from build123d import *
from build123d.topology import SkipClean

# Parameters (mm, degrees)
SKETCH1_R               = 107.5
BOSS_EXTRUDE1_DEPTH     = 5
BOSS_EXTRUDE2_DEPTH     = 70
CUT_EXTRUDE2_DEPTH      = 10
CUT_EXTRUDE2_DEPTH_BACK = 10
BOSS_EXTRUDE4_DEPTH     = 55
CUT_EXTRUDE3_DEPTH      = 10
CUT_EXTRUDE3_DEPTH_BACK = 10
CUT_EXTRUDE4_DEPTH      = 10
CUT_EXTRUDE4_DEPTH_BACK = 10
CUT_EXTRUDE5_DEPTH      = 80
CUT_EXTRUDE6_START      = -10
CUT_EXTRUDE6_DEPTH      = 10


with BuildPart() as part:
    # Sketch1 → Boss-Extrude1 (new body)
    with BuildSketch(Plane(origin=(0, 0, 0), x_dir=(1, 0, 0), z_dir=(0, 1, 0))):
        with Locations(Location((0, 0, 0), (0, 0, 270))):
            Circle(SKETCH1_R)
    extrude(amount=BOSS_EXTRUDE1_DEPTH)

    # Sketch2 → Boss-Extrude2 (add)
    with SkipClean():  # the faces are left unmerged after this step: merging them gives an invalid solid
        with BuildSketch(Plane(origin=(0, 5, 0), x_dir=(1, 0, 0), z_dir=(0, 1, 0))):
            with BuildLine():
                Line((-9.756097561, 99.522954942), (-9.756097561, 107.056380288))
                ThreePointArc((-9.756097561, 107.056380288), (-93.036435814, 53.856026692), (-97.694053207, -44.856682534))
                Line((-97.694053207, -44.856682534), (-91.168439698, -41.089117817))
                ThreePointArc((-91.168439698, -41.089117817), (-86.541200053, 50.106094373), (-9.756097561, 99.522954942))
            make_face()
            with BuildLine():
                Line((10, 99.498743711), (10, 107.033873143))
                ThreePointArc((10, 107.033873143), (93.158905169, 53.643903547), (97.591593747, -45.079161814))
                Line((97.591593747, -45.079161814), (91.06745602, -41.312449141))
                ThreePointArc((91.06745602, -41.312449141), (86.663750638, 49.893830534), (10, 99.498743711))
            make_face()
            with BuildLine():
                Line((81.168439698, -58.409625893), (87.694053207, -62.177190609))
                ThreePointArc((87.694053207, -62.177190609), (-0.122469355, -107.499930238), (-87.835496186, -61.977218474))
                Line((-87.835496186, -61.977218474), (-81.311358459, -58.210505801))
                ThreePointArc((-81.311358459, -58.210505801), (-0.122550585, -99.999924907), (81.168439698, -58.409625893))
            make_face()
        extrude(amount=BOSS_EXTRUDE2_DEPTH)

    # Sketch4 → Cut-Extrude2 (cut, two sides: drawn at the far end of the back side and taken through both)
    with SkipClean():  # the faces are left unmerged after this step: merging them gives an invalid solid
        with BuildSketch(Plane.ZY.offset(107.5).offset(-CUT_EXTRUDE2_DEPTH_BACK)):
            with BuildLine():
                Line((-1.48492424, 71.48492424), (0, 72.969848481))
                Line((0, 72.969848481), (1.48492424, 71.48492424))
                ThreePointArc((1.48492424, 71.48492424), (0, 67.9), (-1.48492424, 71.48492424))
            make_face()
        extrude(amount=CUT_EXTRUDE2_DEPTH + CUT_EXTRUDE2_DEPTH_BACK, mode=Mode.SUBTRACT)

    # Sketch6 → Boss-Extrude4 (add)
    with SkipClean():  # the faces are left unmerged after this step: merging them gives an invalid solid
        with BuildSketch(Plane(origin=(0, 5, 0), x_dir=(1, 0, 0), z_dir=(0, 1, 0))):
            with BuildLine():
                Line((94.638496319, 8.279795561), (99.619469809, 8.715574275))
                ThreePointArc((99.619469809, 8.715574275), (100, 0), (99.619469809, -8.715574275))
                Line((99.619469809, -8.715574275), (94.638496319, -8.279795561))
                ThreePointArc((94.638496319, -8.279795561), (95, 0), (94.638496319, 8.279795561))
            make_face()
            with BuildLine():
                Line((54.489761453, -77.819444207), (57.357643635, -81.915204429))
                ThreePointArc((57.357643635, -81.915204429), (50, -86.602540378), (42.261826174, -90.630778704))
                Line((42.261826174, -90.630778704), (40.148734865, -86.099239768))
                ThreePointArc((40.148734865, -86.099239768), (47.5, -82.27241336), (54.489761453, -77.819444207))
            make_face()
            with BuildLine():
                Line((-40.148734865, -86.099239768), (-42.261826174, -90.630778704))
                ThreePointArc((-42.261826174, -90.630778704), (-50, -86.602540378), (-57.357643635, -81.915204429))
                Line((-57.357643635, -81.915204429), (-54.489761453, -77.819444207))
                ThreePointArc((-54.489761453, -77.819444207), (-47.5, -82.27241336), (-40.148734865, -86.099239768))
            make_face()
            with BuildLine():
                Line((-94.638496319, -8.279795561), (-99.619469809, -8.715574275))
                ThreePointArc((-99.619469809, -8.715574275), (-100, 0), (-99.619469809, 8.715574275))
                Line((-99.619469809, 8.715574275), (-94.638496319, 8.279795561))
                ThreePointArc((-94.638496319, 8.279795561), (-95, 0), (-94.638496319, -8.279795561))
            make_face()
            with BuildLine():
                Line((-54.489761453, 77.819444207), (-57.357643635, 81.915204429))
                ThreePointArc((-57.357643635, 81.915204429), (-50, 86.602540378), (-42.261826174, 90.630778704))
                Line((-42.261826174, 90.630778704), (-40.148734865, 86.099239768))
                ThreePointArc((-40.148734865, 86.099239768), (-47.5, 82.27241336), (-54.489761453, 77.819444207))
            make_face()
            with BuildLine():
                Line((40.148734865, 86.099239768), (42.261826174, 90.630778704))
                ThreePointArc((42.261826174, 90.630778704), (50, 86.602540378), (57.357643635, 81.915204429))
                Line((57.357643635, 81.915204429), (54.489761453, 77.819444207))
                ThreePointArc((54.489761453, 77.819444207), (47.5, 82.27241336), (40.148734865, 86.099239768))
            make_face()
        extrude(amount=BOSS_EXTRUDE4_DEPTH)

    # Sketch7 → Cut-Extrude3 (cut, two sides: drawn at the far end of the back side and taken through both)
    with SkipClean():  # the faces are left unmerged after this step: merging them gives an invalid solid
        with BuildSketch(Plane(origin=(53.75, 0, 93.097730907), x_dir=(0.8660254037844344, 0, -0.5000000000000075), z_dir=(0.5000000000000075, 0, 0.8660254037844344)).offset(-CUT_EXTRUDE3_DEPTH_BACK)):
            with BuildLine():
                Line((0, 72.969848481), (-1.48492424, 71.48492424))
                ThreePointArc((-1.48492424, 71.48492424), (0, 67.9), (1.48492424, 71.48492424))
                Line((1.48492424, 71.48492424), (0, 72.969848481))
            make_face()
        extrude(amount=CUT_EXTRUDE3_DEPTH + CUT_EXTRUDE3_DEPTH_BACK, mode=Mode.SUBTRACT)

    # Sketch8 → Cut-Extrude4 (cut, two sides: drawn at the far end of the back side and taken through both)
    with SkipClean():  # the faces are left unmerged after this step: merging them gives an invalid solid
        with BuildSketch(Plane(origin=(53.75, 0, -93.097730907), x_dir=(-0.8660254037844379, 0, -0.5000000000000013), z_dir=(0.5000000000000012, 0, -0.8660254037844378)).offset(-CUT_EXTRUDE4_DEPTH_BACK)):
            with BuildLine():
                Line((-1.48492424, 71.48492424), (0, 72.969848481))
                Line((0, 72.969848481), (1.48492424, 71.48492424))
                ThreePointArc((1.48492424, 71.48492424), (0, 67.9), (-1.48492424, 71.48492424))
            make_face()
        extrude(amount=CUT_EXTRUDE4_DEPTH + CUT_EXTRUDE4_DEPTH_BACK, mode=Mode.SUBTRACT)

    # Sketch10 → Cut-Extrude5 (cut)
    with SkipClean():  # the faces are left unmerged after this step: merging them gives an invalid solid
        with BuildSketch(Plane(origin=(0, 5, 0), x_dir=(1, 0, 0), z_dir=(0, 1, 0))):
            with BuildLine():
                Line((-34.309046601, -93.930236459), (-36.882225096, -100.975004194))
                ThreePointArc((-36.882225096, -100.975004194), (-0.122469355, -107.499930238), (36.652057999, -101.058778166))
                Line((36.652057999, -101.058778166), (34.094937673, -94.008165736))
                ThreePointArc((34.094937673, -94.008165736), (-0.113924981, -99.999935105), (-34.309046601, -93.930236459))
            make_face()
            with BuildLine():
                Line((-64.191447657, 76.677624166), (-69.005806231, 82.428445979))
                ThreePointArc((-69.005806231, 82.428445979), (-93.036435814, 53.856026692), (-105.845498167, 18.787775755))
                Line((-105.845498167, 18.787775755), (-98.460928527, 17.477000703))
                ThreePointArc((-98.460928527, 17.477000703), (-86.545521688, 50.09862948), (-64.191447657, 76.677624166))
            make_face()
            with BuildLine():
                Line((98.500494258, 17.252612293), (105.888031327, 18.546558215))
                ThreePointArc((105.888031327, 18.546558215), (93.158905169, 53.643903547), (69.193440168, 82.271002411))
                Line((69.193440168, 82.271002411), (64.365990854, 76.531165034))
                ThreePointArc((64.365990854, 76.531165034), (86.659446669, 49.901305625), (98.500494258, 17.252612293))
            make_face()
        extrude(amount=CUT_EXTRUDE5_DEPTH, mode=Mode.SUBTRACT)

    # Sketch11 → Cut-Extrude6 (cut)
    with SkipClean():  # the faces are left unmerged after this step: merging them gives an invalid solid
        with BuildSketch(Plane(origin=(0, 75, 0), x_dir=(1, 0, 0), z_dir=(0, 1, 0)).offset(CUT_EXTRUDE6_START)):
            with BuildLine():
                Line((-64.191447657, 76.677624166), (-69.005806231, 82.428445979))
                ThreePointArc((-69.005806231, 82.428445979), (-41.261279177, 99.266091092), (-9.756097561, 107.056380288))
                Line((-9.756097561, 107.056380288), (-9.075439592, 99.587330501))
                ThreePointArc((-9.075439592, 99.587330501), (-38.382585281, 92.340549853), (-64.191447657, 76.677624166))
            make_face()
            with BuildLine():
                Line((98.500494258, 17.252612293), (105.888031327, 18.546558215))
                ThreePointArc((105.888031327, 18.546558215), (106.597596209, -13.899729586), (97.591593747, -45.079161814))
                Line((97.591593747, -45.079161814), (90.782877904, -41.934104013))
                ThreePointArc((90.782877904, -41.934104013), (99.160554613, -12.92998101), (98.500494258, 17.252612293))
            make_face()
            with BuildLine():
                Line((-34.309046601, -93.930236459), (-36.882225096, -100.975004194))
                ThreePointArc((-36.882225096, -100.975004194), (-65.336317032, -85.366361506), (-87.835496186, -61.977218474))
                Line((-87.835496186, -61.977218474), (-81.707438313, -57.653226487))
                ThreePointArc((-81.707438313, -57.653226487), (-60.777969332, -79.410568843), (-34.309046601, -93.930236459))
            make_face()
        extrude(amount=CUT_EXTRUDE6_DEPTH, mode=Mode.SUBTRACT)


solid = part.part
The model under review builds one solid part; all positions refer to its coordinate system, in mm. A direction names the side the tool comes from. Round coordinates to 2 decimals unless told otherwise and drop trailing zeros. Loops run counter-clockwise (first coordinate to the right, second up) from the corner with the lowest first, then second, coordinate; pieces in that order, holes last. Notation, with made-up numbers: (-9, 35.25) -> (47, 35.25) arc R11 cw to (47, 44.25) -> close; hole circle Ø8 at (-3, -6). An arc over 180 degrees is marked (long way). Write item = value, one per line. Start each with the question number.
Item 1: Take a section at C-C on x = -75. Give the boundary of the cut face in (y, z).
Item 2: Take a section at A-A on y = 9. Count the separate pieces of the cut face and the enclosed holes in it, plus the area to 3 significant figures.
Item 3: Take a section at B-B on z = 35. Give the boundary of the cut face in (x, y), plus the area to 3 significant figures.
Item 4: Take a section at D-D on x = 0. Give the boundary of the cut face in (y, z), plus the area to 4 significant figures.
Item 5: To check wall thickness, follow L1, parallel to Y at x = -105, z = 0; L2, parallel to Y at x = -93.5, z = 29; L3, parallel to X at y = 28, z = 24. State the ranges of each line that lie inside material, in increasing order.
Item 6: Mouldability with a two-part tool opening along Y and no side actions: class faces 5 (the flat face through (52.498, 72.217, -89.423)), 6 (the flat face through (-49, 60, 84)), 7 (the cylindrical face through (47.4, 32.11, 82.33)) as released by +Y, released by -Y, zero draft, split by the parting line, or undercut.
Item 7: Insertion check: pin 1 (4 mm diameter, centred on x = -44.5, z = -81.5, fed in from +Y); pin 2 (2 mm diameter, centred on x = 23.5, y = 50.5, fed in from +Z); pin 3 (3 mm diameter, centred on y = 39.5, z = -78, fed in from +X). Each pin has a flat end and moves straight along its axis. Give the tip position at first contact, or say it passes through.
Item 8: For faces 1 (the flat face through (-94.48, 39.51, 43)), 2 (the flat face through (102.14, 34.58, -17.89)), 3 (the flat face through (66.81, 39.51, -79.44)), 4 (the flat face through (-97.16, 32.11, -8.5)), list the 3-axis set-ups (+Z, -Z, +X, -X, +Y, -Y) from which the entire face can be reached by the end or side of a thin tool; tool diameter is ignored.
Result:
q1.outline = (0, -77.01) -> (5, -77.01) -> (5, 66.14) -> (65, 66.14) -> (65, 77.01) -> (0, 77.01) -> close
q2.separate_pieces = 6
q2.enclosed_holes = 0
q2.area = 3,320 mm²
q3.outline = (-101.64, 0) -> (101.64, 0) -> (101.64, 65) -> (93.67, 65) -> (93.67, 5) -> (-93.67, 5) -> (-93.67, 75) -> (-101.64, 75) -> close
q3.area = 2,050 mm²
q4.outline = (0, -107.5) -> (5, -107.5) -> (5, 107.5) -> (0, 107.5) -> close
q4.area = 1,075 mm²
q5.L1 = 0 to 67.9, 72.97 to 75
q5.L2 = 0 to 5
q5.L3 = -104.79 to -97.08, 97.08 to 104.79
q6.face_5 = undercut
q6.face_6 = released by +Y
q6.face_7 = zero draft
q7.pin_1 = 5
q7.pin_2 = -96.95
q7.pin_3 = 66.86
q8.face_1 = +Z, +Y
q8.face_2 = -Z, +Y
q8.face_3 = +X, +Y
q8.face_4 = +Y
